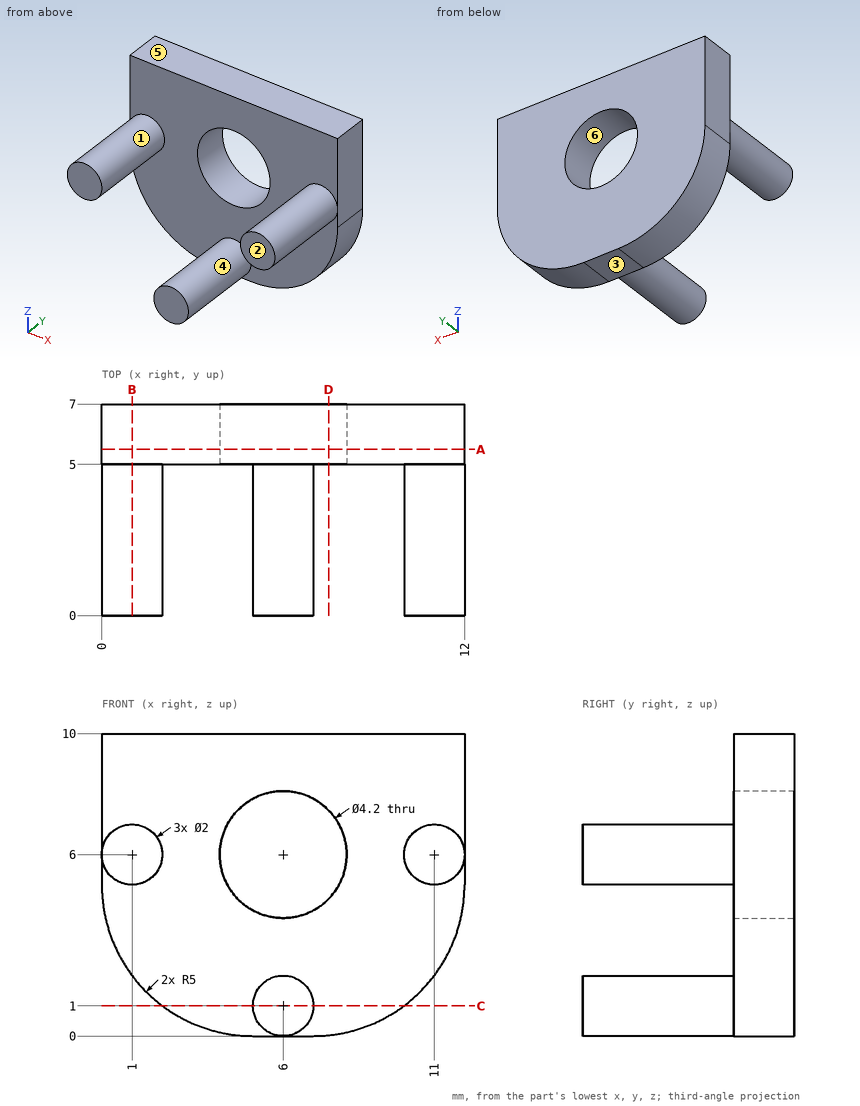
Check sheet for the drawn part. Datum: minimum x, y, z corner. Units: mm. A direction names the side the tool comes from. Give positions to 0.01 mm unless a question says otherwise; leave off trailing zeros. Write each loop counter-clockwise with the first axis right and the second up, starting at its lowest first coordinate (ties: lowest second). Pieces come first, ordered by that corner, then holes. Notation, with made-up numbers: (11.5, 79) -> (20.5, 79) arc R28 ccw to (20.5, 105) -> close; hole circle Ø6 at (-39.75, 27.25). An arc over 180 degrees is marked (long way). Use one line per item in the form item = value. Start each with the question number.
1. Access from +Z, -Z, +X, -X, +Y, -Y to the whole of each face (thin tool, end or side, straight path). Record for the marked faces 1 and 2.
2. Section check B-B (x = 1). Record the cut outline in (y, z).
3. Thickness scan on line 1 along X through (y, z) = (5.5, 6); line 2 along X through (y, z) = (4.25, 6); line 3 along Y through (x, z) = (8.25, 5). Record the ranges inside material, lowest first. Write a range as from..to.
4. Section check A-A (y = 5.5). Record the cut outline in (x, z).
5. Go/stop test with a flat-tipped pin: P1, Ø1, axis at y = 1.5, z = 1.5, coming from the +X side. Record where the tip stops, or that it passes through.
6. Section check D-D (x = 7.5). Record the cut outline in (y, z).
7. Mould release check, pull along Z, two halves, no side actions. Record for the marked faces 3, 4, 5 and 6: pulls with the +Z half, pulls with the -Z half, needs draft (parallel to the pull), parting line crosses it, or undercut.
8. Section check C-C (z = 1). Record the cut outline in (x, y).
Conclusion:
q1.face_1 = -Y
q1.face_2 = +Z, -Z, +X, -X, -Y
q2.outline = (0, 5) -> (5, 5) -> (5, 2) -> (7, 2) -> (7, 10) -> (5, 10) -> (5, 7) -> (0, 7) -> close
q3.line_1 = 0..3.9, 8.1..12
q3.line_2 = 0..2, 10..12
q3.line_3 = 5..7
q4.outline = (0, 5) arc R5 ccw to (5, 0) -> (7, 0) arc R5 ccw to (12, 5) -> (12, 10) -> (0, 10) -> close; hole circle Ø4.2 at (6, 6)
q5.P1 = 7
q6.outline = (5, 0.03) -> (7, 0.03) -> (7, 4.53) -> (5, 4.53) -> close; (5, 7.47) -> (7, 7.47) -> (7, 10) -> (5, 10) -> close
q7.face_3 = pulls with the -Z half
q7.face_4 = parting line crosses it
q7.face_5 = pulls with the +Z half
q7.face_6 = undercut
q8.outline = (2, 5) -> (5, 5) -> (5, 0) -> (7, 0) -> (7, 5) -> (10, 5) -> (10, 7) -> (2, 7) -> close
